The listing builds one solid part. Answer for the finished solid, in the listing's coordinates (mm). A direction names the side the tool comes from. Give positions to 0.01 mm unless a question says otherwise; leave off trailing zeros. Loops run counter-clockwise (first coordinate to the right, second up) from the corner with the lowest first, then second, coordinate; pieces in that order, holes last. Notation, with made-up numbers: (68.25, 20) - (82.25, 20) arc R18 ccw to (82.25, 32) - close; hole circle Ø2 at (56.25, 85.5). An arc over 180 degrees is marked (long way). Answer as CSV lines item,"result". Start each with the question number.
1) For faces 1 (the face through (0, 31, -11.8)), 2 (the face through (0, 30, -12.7)), determine the directions among +Z, -Z, +X, -X, +Y, -Y from which every point of the face is accessible in a straight line to the end or side of a thin tool.
2) A cutting plane is placed at A-A (x = 0). Determine the outline of the cut face in (y, z).
3) A cutting plane is placed at D-D (x = -6.5). Determine the outline of the cut face in (y, z).
4) For a pull along Z with two mould halves and no side action, classify faces 3 (the face through (-12.7, 25, 0)), 4 (the face through (11.8, 26, 0)), 5 (the face through (0, 30, 12.7)) as pulls with the +Z half, pulls with the -Z half, needs draft (parallel to the pull), parting line crosses it, or undercut.
5) A cutting plane is placed at C-C (y = 38.5). Determine the outline of the cut face in (x, z).
6) Find the intervals of material crossed by line 1 along X through (y, z) = (11, -3.25), in increasing order.
7) A cutting plane is placed at B-B (z = 0). Determine the outline of the cut face in (x, y), and give its area (3 significant figures).
```python
from build123d import *

# Parameters (mm, degrees)
SKETCH1_W           = 25.4
SKETCH1_H           = 25.4
SKETCH1_W_2         = 23.6
SKETCH1_H_2         = 23.6
BOSS_EXTRUDE1_DEPTH = 50
CUT_EXTRUDE1_DEPTH  = 25.4


with BuildPart() as part:
    # Sketch1 → Boss-Extrude1 (new body)
    with BuildSketch(Plane(origin=(0, 0, 0), x_dir=(1, 0, 0), z_dir=(0, 1, 0))):
        Rectangle(SKETCH1_W, SKETCH1_H)
        Rectangle(SKETCH1_W_2, SKETCH1_H_2, mode=Mode.SUBTRACT)
    extrude(amount=BOSS_EXTRUDE1_DEPTH)

    # Sketch2 → Cut-Extrude1 (cut)
    with BuildSketch(Plane.XY.offset(12.7)):
        with BuildLine():
            Line((-12, 0), (12, 0))
            ThreePointArc((12, 0), (0, 12), (-12, 0))
        make_face()
    extrude(amount=-CUT_EXTRUDE1_DEPTH, mode=Mode.SUBTRACT)


solid = part.part
```
Ans:
1,face 1,"+Y, -Y"
1,face 2,"-Z, +X, -X, +Y, -Y"
2,outline,"(12, -12.7) - (50, -12.7) - (50, -11.8) - (12, -11.8) - close; (12, 11.8) - (50, 11.8) - (50, 12.7) - (12, 12.7) - close"
3,outline,"(10.09, -12.7) - (50, -12.7) - (50, -11.8) - (10.09, -11.8) - close; (10.09, 11.8) - (50, 11.8) - (50, 12.7) - (10.09, 12.7) - close"
4,face 3,"needs draft"
4,face 4,"undercut"
4,face 5,"pulls with the +Z half"
5,outline,"(-12.7, -12.7) - (12.7, -12.7) - (12.7, 12.7) - (-12.7, 12.7) - close; hole (-11.8, -11.8) - (11.8, -11.8) - (11.8, 11.8) - (-11.8, 11.8) - close"
6,line 1,"-12.7 to -11.8, 11.8 to 12.7"
7,outline,"(-12.7, 0) - (-12, 0) arc R12 cw to (-11.8, 2.18) - (-11.8, 50) - (-12.7, 50) - close; (11.8, 2.18) arc R12 cw to (12, 0) - (12.7, 0) - (12.7, 50) - (11.8, 50) - close"
7,area,"89.4 mm2"
